The model under review builds one solid part; all positions refer to its coordinate system, in mm. Round coordinates to 2 decimals unless told otherwise and drop trailing zeros. Write each loop counter-clockwise with the first axis right and the second up, starting at its lowest first coordinate (ties: lowest second). Pieces come first, ordered by that corner, then holes. Notation, with made-up numbers: (50.5, 62) -> (89.5, 62) arc R21 ccw to (89.5, 84) -> close; hole circle Ø4 at (-9, -25.5). An arc over 180 degrees is marked (long way). Return JSON: item names as keys, results as strings. Group by question number.
1. Take a section at B-B, the plane y = -7. Write out the cut boundary in (x, z) (3 decimals).
2. For line 1 along Y through (x, z) = (-38.5, -2.6); line 2 along Y through (x, z) = (-57, -1.6); line 3 along Y through (x, z) = (-41.5, -1), list the stretches that pass through material, from the lowest coordinate up. Write a range as from..to.
3. Take a section at C-C, the plane x = -25.4. Write out the cut boundary in (y, z) (3 decimals).
4. Clearance check with a flat-ended pin moving along its axis: P1, Ø9, axis at x = 0, y = 81.84, coming from the -Z side. State where the tip first meets the part, or that it passes through.
5. Take a section at A-A, the plane x = 0. Write out the cut boundary in (y, z) (1 decimal).
6. Take a section at D-D, the plane z = -1.45. Give the number of separate pieces and of enclosed holes in the cut face, then the cut area to 3 significant figures.
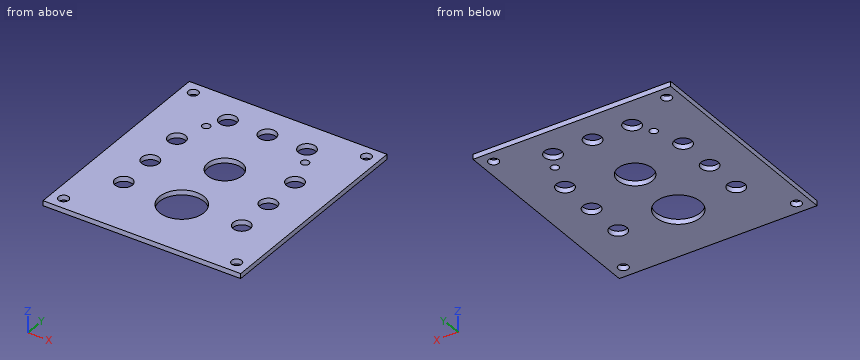
from build123d import *

# Parameters (mm, degrees)
SKETCH1_W           = 127
SKETCH1_H           = 139.7
SKETCH1_R           = 3.2512
SKETCH1_R_2         = 5.5626
SKETCH1_R_3         = 11.1125
SKETCH1_R_4         = 14.2875
SKETCH1_R_5         = 2.54
BOSS_EXTRUDE1_DEPTH = 3.175


with BuildPart() as part:
    # Sketch1 → Boss-Extrude1 (new body)
    with BuildSketch(Plane(origin=(0, 0, -3.175), x_dir=(-1, 0, 0), z_dir=(0, 0, -1))):
        with Locations((0, 31.75)):
            Rectangle(SKETCH1_W, SKETCH1_H)
        with Locations((55.5752, -30.1752)):
            Circle(SKETCH1_R, mode=Mode.SUBTRACT)
        with Locations((0, 81.8388)):
            Circle(SKETCH1_R_2, mode=Mode.SUBTRACT)
        with Locations((37.915221739, 51.777178589)):
            Circle(SKETCH1_R_2, mode=Mode.SUBTRACT)
        with Locations((-37.915221739, 0.977178589)):
            Circle(SKETCH1_R_2, mode=Mode.SUBTRACT)
        with Locations((-25.4, 81.8388)):
            Circle(SKETCH1_R_2, mode=Mode.SUBTRACT)
        with Locations((0, 41.148)):
            Circle(SKETCH1_R_3, mode=Mode.SUBTRACT)
        with Locations((-55.5752, 93.6752)):
            Circle(SKETCH1_R, mode=Mode.SUBTRACT)
        with Locations((-55.5752, -30.1752)):
            Circle(SKETCH1_R, mode=Mode.SUBTRACT)
        with Locations((55.5752, 93.6752)):
            Circle(SKETCH1_R, mode=Mode.SUBTRACT)
        Circle(SKETCH1_R_4, mode=Mode.SUBTRACT)
        with Locations((25.4, 81.8388)):
            Circle(SKETCH1_R_2, mode=Mode.SUBTRACT)
        with Locations((-37.915221739, 51.777178589)):
            Circle(SKETCH1_R_2, mode=Mode.SUBTRACT)
        with Locations((37.915221739, 0.977178589)):
            Circle(SKETCH1_R_2, mode=Mode.SUBTRACT)
        with Locations((37.915221739, 26.377178589)):
            Circle(SKETCH1_R_2, mode=Mode.SUBTRACT)
        with Locations((-37.915221739, 26.377178589)):
            Circle(SKETCH1_R_2, mode=Mode.SUBTRACT)
        with Locations((31.75, 70.58025)):
            Circle(SKETCH1_R_5, mode=Mode.SUBTRACT)
        with Locations((-31.75, 70.58025)):
            Circle(SKETCH1_R_5, mode=Mode.SUBTRACT)
    extrude(amount=-BOSS_EXTRUDE1_DEPTH)


solid = part.part
Output:
{
 "1": {"outline": "(-63.5, -3.175) -> (-12.455, -3.175) -> (-12.455, 0) -> (-63.5, 0) -> close; (12.455, -3.175) -> (63.5, -3.175) -> (63.5, 0) -> (12.455, 0) -> close"},
 "2": {"line 1": "y = -38.1..-4.55, 6.51..20.85, 31.91..46.25, 57.31..101.6", "line 2": "y = -38.1..-33.1, -27.25..90.75, 96.6..101.6", "line 3": "y = -38.1..-3.28, 5.23..22.12, 30.63..47.52, 56.03..101.6"},
 "3": {"outline": "(-38.1, -3.175) -> (76.276, -3.175) -> (76.276, 0) -> (-38.1, 0) -> close; (87.401, -3.175) -> (101.6, -3.175) -> (101.6, 0) -> (87.401, 0) -> close"},
 "4": {"P1": "passes through"},
 "5": {"outline": "(-38.1, -3.2) -> (-14.3, -3.2) -> (-14.3, 0) -> (-38.1, 0) -> close; (14.3, -3.2) -> (30, -3.2) -> (30, 0) -> (14.3, 0) -> close; (52.3, -3.2) -> (76.3, -3.2) -> (76.3, 0) -> (52.3, 0) -> close; (87.4, -3.2) -> (101.6, -3.2) -> (101.6, 0) -> (87.4, 0) -> close"},
 "6": {"separate pieces": "1", "enclosed holes": "17", "area": "15,700 mm^2"}
}
